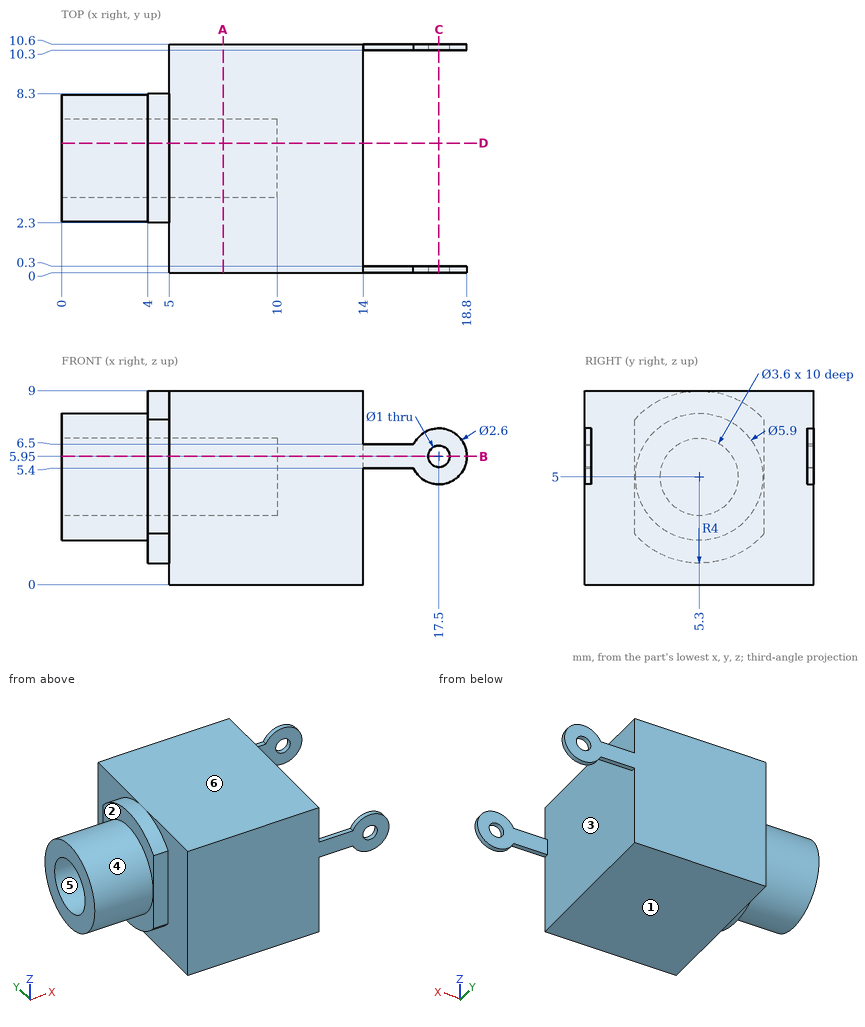
Source: three-view drawing plus pictorial views. Frame: mm from the lowest corner of the part. A direction names the side the tool comes from. Coordinates: 2 decimals unless noted, no trailing zeros. Loops run counter-clockwise (first coordinate to the right, second up) from the corner with the lowest first, then second, coordinate; pieces in that order, holes last. Notation, with made-up numbers: (56, 49) -> (74, 49) arc R36 ccw to (74, 86) -> close; hole circle Ø7 at (-11, -16.5). An arc over 180 degrees is marked (long way). One line per item, written item: value.
(1) Ray query, line 1 along Z through (x, y) = (6.75, 5.3); line 2 along Z through (x, y) = (17.5, 0.25); line 3 along X through (y, z) = (9, 8.75). Return the intervals inside material, ascending.
Answer below:
line 1: z = 0 to 3.2, 6.8 to 9
line 2: z = 4.65 to 5.45, 6.45 to 7.25
line 3: x = 5 to 14
(2) Cut plane A-A (x = 7.5). Output: boundary loops of the cut face in (y, z).
Answer below:
outline: (0, 0) -> (10.6, 0) -> (10.6, 9) -> (0, 9) -> close; hole circle Ø3.6 at (5.3, 5)
(3) Cut plane B-B (z = 5.95). Output: boundary loops of the cut face in (x, y), then the cut area to 3 significant figures.
Answer below:
outline: (0, 2.51) -> (4, 2.51) -> (4, 2.3) -> (5, 2.3) -> (5, 0) -> (17, 0) -> (17, 0.3) -> (14, 0.3) -> (14, 10.3) -> (17, 10.3) -> (17, 10.6) -> (5, 10.6) -> (5, 8.3) -> (4, 8.3) -> (4, 8.09) -> (0, 8.09) -> (0, 6.83) -> (10, 6.83) -> (10, 3.77) -> (0, 3.77) -> close; (18, 0) -> (18.8, 0) -> (18.8, 0.3) -> (18, 0.3) -> close; (18, 10.3) -> (18.8, 10.3) -> (18.8, 10.6) -> (18, 10.6) -> close
area: 95.4 mm2
(4) Pin query (flat end, axial travel): pin 1 Ø1.5 at (x, y) = (2.5, 5) entering from -Z; pin 2 Ø2.5 at (y, z) = (7.5, 5) entering from +X; pin 3 Ø3 at (x, z) = (3, 1.5) entering from +Y. Return the tip coordinate at first contact, or that it passes through.
Answer below:
pin 1: stops at z = 2.05
pin 2: stops at x = 14
pin 3: stops at y = 8.3
(5) Set-up query: the marked faces 1 and 2. Return all of +Z, -Z, +X, -X, +Y, -Y with unobstructed straight access to the full face (end or side cutting, diameter ignored); none if empty.
Answer below:
face 1: -Z, +X, -X, +Y, -Y
face 2: +Z, -X
(6) Cut plane D-D (y = 6). Output: boundary loops of the cut face in (x, z).
Answer below:
outline: (0, 2.13) -> (4, 2.13) -> (4, 1.06) -> (5, 1.06) -> (5, 0) -> (14, 0) -> (14, 9) -> (5, 9) -> (5, 8.94) -> (4, 8.94) -> (4, 7.87) -> (0, 7.87) -> (0, 6.66) -> (10, 6.66) -> (10, 3.34) -> (0, 3.34) -> close
(7) Draft query along Z for the marked faces 3, 4, 5 and 6. Return one class per face: pulls with the +Z half, pulls with the -Z half, needs draft (parallel to the pull), parting line crosses it, or undercut.
Answer below:
face 3: needs draft
face 4: parting line crosses it
face 5: undercut
face 6: pulls with the +Z half
(8) Cut plane C-C (x = 17.5). Output: boundary loops of the cut face in (y, z), then the cut area to 3 significant figures.
Answer below:
outline: (0, 4.65) -> (0.3, 4.65) -> (0.3, 5.45) -> (0, 5.45) -> close; (0, 6.45) -> (0.3, 6.45) -> (0.3, 7.25) -> (0, 7.25) -> close; (10.3, 4.65) -> (10.6, 4.65) -> (10.6, 5.45) -> (10.3, 5.45) -> close; (10.3, 6.45) -> (10.6, 6.45) -> (10.6, 7.25) -> (10.3, 7.25) -> close
area: 0.960 mm2
